Read the model definition and answer for the solid it produces. Units are mm, in the model's axes. A direction names the side the tool comes from. Coordinates: 2 decimals unless noted, no trailing zeros. Loops run counter-clockwise (first coordinate to the right, second up) from the corner with the lowest first, then second, coordinate; pieces in that order, holes last. Notation, with made-up numbers: (-0.75, 75) - (58.25, 75) arc R12 ccw to (58.25, 97) - close; hole circle Ø9 at (3, -28). An arc over 180 degrees is marked (long way). Use CSV: the item, a comma, the result in double quotes.
```python
from build123d import *

# Parameters (mm, degrees)
F1_DEPTH = 63.5
F0_W     = 25.4
F0_H     = 19.05
F2_DEPTH = 25.4
F3_DEPTH = 7.9375
F5_R     = 5.08


with BuildPart() as f1:
    # F0 (on Front) → F1 (new body, symmetric)
    with BuildSketch(Plane.XZ):
        Polygon((-41.275, 9.525), (-41.275, -9.525), (41.275, -9.525), (41.275, 9.525), (22.225, 9.525), align=None)
    extrude(amount=F1_DEPTH, both=True)

    # F0 (on Front) → F2 (join, symmetric)
    with BuildSketch(Plane.XZ):
        with Locations((73.025, 52.4002)):
            Rectangle(F0_W, F0_H)
        with BuildLine():
            Line((22.225, 9.525), (41.275, 9.525))
            Line((41.275, 9.525), (41.275, 27.0002))
            ThreePointArc((41.275, 27.0002), (45.9246798487, 38.2255201513), (57.15, 42.8752))
            Line((57.15, 42.8752), (60.325, 42.8752))
            Line((60.325, 42.8752), (60.325, 61.9252))
            Line((60.325, 61.9252), (57.15, 61.9252))
            add(Edge.make_bspline(
                [(55.6078581678, 61.8911361234), (56.1258190219, 61.9074850682), (56.63993318, 61.918866137), (57.15, 61.9252)],
                knots=[110.0024937652, 110.0024937652, 110.0024937652, 110.0024937652, 111.5045361635, 111.5045361635, 111.5045361635, 111.5045361635], degree=3))
            ThreePointArc((55.6078581678, 61.8911361234), (31.9149556322, 51.1445194304), (22.225, 27.0002))
            Line((22.225, 27.0002), (22.225, 9.525))
        make_face()
    extrude(amount=F2_DEPTH, both=True)

    # F0 (on Front) → F3 (join, symmetric)
    with BuildSketch(Plane.XZ):
        with BuildLine():
            add(Edge.make_bspline(
                [(-41.275, 9.525), (-40.8895493479, 32.8517610266), (17.6748506275, 60.6938165945), (55.6078581678, 61.8911361234)],
                knots=[0, 0, 0, 0, 110.0024937652, 110.0024937652, 110.0024937652, 110.0024937652], degree=3))
            Line((-41.275, 9.525), (22.225, 9.525))
            Line((22.225, 9.525), (22.225, 27.0002))
            ThreePointArc((22.225, 27.0002), (31.9149556322, 51.1445194304), (55.6078581678, 61.8911361234))
        make_face()
    extrude(amount=F3_DEPTH, both=True)

    # F0 (on Front) → F4 (revolve)
    with BuildSketch(Plane.XZ):
        Polygon((85.725, 66.675), (85.725, 61.9252), (85.725, 42.8752), (85.725, 38.1), (111.125, 38.1), (111.125, 66.675), align=None)
    revolve(axis=Axis((85.725, 0, 52.3875), (0, 0, 1)))

    # F5
    f5_edges = [f1.edges().sort_by_distance(p)[0] for p in [
        (41.275, -63.5, 0),
        (-41.275, -63.5, 0),
        (-41.275, 63.5, 0),
        (41.275, 63.5, 0),
    ]]
    fillet(f5_edges, radius=F5_R)


solid = f1.part
```
Q1. A tool of negligible diameter and unlimited length cuts with its end or side. For faces 1 (the face through (45.8, -0.4, 38.1)), 2 (the face through (22.225, -17, 18)), 3 (the face through (60, -2, 61.925)), from which of +Z, -Z, +X, -X, +Y, -Y can it reach the whole face along a straight path? Write none if from no direction.
Reported:
face 1,"-Z, +Y, -Y"
face 2,"+Z, -X, -Y"
face 3,"+Z, -X"
Q2. Given P1, Ø5, axis at y = 9, z = 10.5, coming from the +X side (3 decimals); P2, Ø8, axis at y = -14, z = 36, coming from the -X side; P3, Ø10, axis at y = -4, z = 30, coming from the -X side, each flat-ended and moving along its own axis, determine where each tip first touches the part or whether it passes through.
Reported:
P1,"stops at x = 41.275"
P2,"stops at x = 22.58"
P3,"stops at x = -33.64"
Q3. The part is cut by section A-A on y = -51. Determine the outline of the cut face in (x, z) (3 decimals).
Reported:
outline,"(-41.275, -9.525) - (41.275, -9.525) - (41.275, 9.525) - (-41.275, 9.525) - close"
Q4. For a pull along X with two mould halves and no side action, classify faces 4 (the face through (46, -25.4, 42)), 5 (the face through (32.17, -16.79, 51.41)), 6 (the face through (60, 2, 42.875)) as +X half, -X half, draft (parallel to the pull), parting line (faces both ways), or undercut.
Reported:
face 4,"draft"
face 5,"-X half"
face 6,"undercut"
Q5. Find the intervals of material crossed by probe 1 along Y at (x, z) = (-12, 23.5); probe 2 along Z at (x, y) = (40.5, -55.5) (3 decimals); probe 3 along Y at (x, z) = (72.5, 45), in increasing order. Write a range as [from, to].
Reported:
probe 1,"y = [-7.94, 7.94]"
probe 2,"z = [-9.525, 9.525]"
probe 3,"y = [-25.4, 25.4]"
